from build123d import *

# Parameters (mm, degrees)
SKETCH1_R           = 10
BOSS_EXTRUDE1_DEPTH = 125
CUT_EXTRUDE1_DEPTH  = 105
SKETCH5_R           = 37.5
CUT_EXTRUDE2_DEPTH  = 76


with BuildPart() as part:
    # Sketch1 → Boss-Extrude1 (new body)
    with BuildSketch(Plane(origin=(0, 0, 0), x_dir=(-1, 0, 0), z_dir=(0, -1, 0))):
        with BuildLine():
            Line((-220.847331583, 50), (-145.847331583, 50))
            Line((-145.847331583, 50), (4.152668417, 23.550952894))
            ThreePointArc((4.152668417, 23.550952894), (23.914264304, 0), (4.152668417, -23.550952894))
            Line((4.152668417, -23.550952894), (-145.847331583, -50))
            Line((-145.847331583, -50), (-220.847331583, -50))
            Line((-220.847331583, -50), (-220.847331583, 50))
        make_face()
        Circle(SKETCH1_R, mode=Mode.SUBTRACT)
    extrude(amount=BOSS_EXTRUDE1_DEPTH)

    # Sketch2 → Cut-Extrude1 (cut)
    with BuildSketch(Plane(origin=(0, -125, 0), x_dir=(-1, 0, 0), z_dir=(0, -1, 0))):
        with BuildLine():
            Line((-145.847331583, 50), (-145.847331583, -50))
            Line((-145.847331583, -50), (4.152668417, -23.550952894))
            ThreePointArc((4.152668417, -23.550952894), (23.914264304, 0), (4.152668417, 23.550952894))
            Line((4.152668417, 23.550952894), (-145.847331583, 50))
        make_face()
    extrude(amount=-CUT_EXTRUDE1_DEPTH, mode=Mode.SUBTRACT)

    # Sketch5 → Cut-Extrude2 (cut, through all)
    with BuildSketch(Plane(origin=(145.847331583, 0, 0), x_dir=(0, 0, -1), z_dir=(-1, 0, 0))):
        with Locations((0, 72.5)):
            Circle(SKETCH5_R)
    extrude(amount=-CUT_EXTRUDE2_DEPTH, mode=Mode.SUBTRACT)


solid = part.part
The model under review builds one solid part; all positions refer to its coordinate system, in mm. A direction names the side the tool comes from. Round coordinates to 2 decimals unless told otherwise and drop trailing zeros. Loops run counter-clockwise (first coordinate to the right, second up) from the corner with the lowest first, then second, coordinate; pieces in that order, holes last. Notation, with made-up numbers: M 35,59 L 86,59 A15 cw 86,65 Z; hole C 29,-8.75 d6. An arc over 180 degrees is marked long. Answer as CSV lines item,"result". Start each with the question number.
Item 1: Consider section C-C (x = 0). Write out the cut boundary in (y, z), then the cut area to 3 significant figures.
Item 2: For faces 4 (the face through (183, -62, 50)), 5 (the face through (81, -20, -1)), list the 3-axis set-ups (+Z, -Z, +X, -X, +Y, -Y) from which the entire face can be reached by the end or side of a thin tool; tool diameter is ignored.
Item 3: Consider section B-B (z = 0). Write out the cut boundary in (x, y).
Item 4: Insertion check: P1, Ø12, axis at x = 145.5, y = -60, coming from the -Z side; P2, Ø1.5, axis at y = -31, z = 0, coming from the -X side; P3, Ø12, axis at x = 43, z = -37.5, coming from the -Y side. Each pin has a flat end and moves straight along its axis. Give the tip position at first contact, or say it passes through.
Item 5: Consider section A-A (y = -11). Write out the cut boundary in (x, z), then the cut area to 3 significant figures.
Item 6: Wall thickness on line 1 (X direction, y = -6.5, z = 0); line 2 (Y direction, x = 195, z = 0); line 3 (Z direction, x = 204, y = -72.5): over which ranges is each line inside the solid? List them lowest first. Write a range as [from, to].
Item 7: Mouldability with a two-part tool opening along Z and no side actions: class faces 1 (the face through (182.82, -109.68, 4.88)), 2 (the face through (220.847, -34, 1)), 3 (the face through (69.8, -9.86, 36.59)) as released by +Z, released by -Z, zero draft, split by the parting line, or undercut.
Item 8: Consider section D-D (y = -88). Write out the cut boundary in (x, z), then the cut area to 3 significant figures.
Answer:
1,outline,"M -20,-24.28 L 0,-24.28 L 0,-10 L -20,-10 Z; M -20,10 L 0,10 L 0,24.28 L -20,24.28 Z"
1,area,"571 mm^2"
2,face 4,"+Z, +X, -X, +Y, -Y"
2,face 5,"+Z, -Z, -X, -Y"
3,outline,"M -23.91,-20 L -10,-20 L -10,0 L -23.91,0 Z; M 10,-20 L 145.85,-20 L 145.85,-35 L 220.85,-35 L 220.85,0 L 10,0 Z; M 145.85,-125 L 220.85,-125 L 220.85,-110 L 145.85,-110 Z"
4,P1,"stops at z = -50"
4,P2,"stops at x = 145.85"
4,P3,"stops at y = -20"
5,outline,"M -4.15,-23.55 L 145.85,-50 L 220.85,-50 L 220.85,50 L 145.85,50 L -4.15,23.55 A23.91 ccw Z; hole C 0,0 d20"
5,area,"18,900 mm^2"
6,line 1,"x = [-23.91, -10], [10, 220.85]"
6,line 2,"y = [-125, -110], [-35, 0]"
6,line 3,"z = [-50, -37.5], [37.5, 50]"
7,face 1,"undercut"
7,face 2,"zero draft"
7,face 3,"released by +Z"
8,outline,"M 145.85,-50 L 220.85,-50 L 220.85,-34.15 L 145.85,-34.15 Z; M 145.85,34.15 L 220.85,34.15 L 220.85,50 L 145.85,50 Z"
8,area,"2,380 mm^2"
